```python
from build123d import *

# Parameters (mm, degrees)
F0_W      = 50
F0_H      = 12.5
F1_DEPTH  = 8
F2_DEPTH  = 75
F4_DEPTH  = 8
F7_DEPTH  = 3
F8_DEPTH  = 1
F11_DEPTH = 3
F14_DEPTH = 3
F15_DEPTH = 8
F16_DEPTH = 8
F17_DEPTH = 12.5
F18_DEPTH = 8


# Not quite as in the source:
# - a feature names something its author has since deleted; it is built from what else it names


with BuildPart() as f1:
    # F0 (on Top) → F1 (new body)
    with BuildSketch(Plane.XY):
        Polygon((42.0179491924, -72.7772228311), (84.0358983849, 0), (42.0179491924, 72.7772228311), (-42.0179491924, 72.7772228311), (-84.0358983849, 0), (-42.0179491924, -72.7772228311), align=None)
        with Locations((0, 54.5829171234)):
            Rectangle(F0_W, F0_H, mode=Mode.SUBTRACT)
    extrude(amount=F1_DEPTH)

    # F0 (on Top) → F2 (join)
    with BuildSketch(Plane.XY):
        Polygon((67.6939940411, -34.3050086158), (87.5, 0), (84.0358983849, 0), (42.0179491924, -72.7772228311), (-42.0179491924, -72.7772228311), (-84.0358983849, 0), (-87.5, 0), (-43.75, -75.7772228311), (43.75, -75.7772228311), (63.1939940411, -42.0992372499), align=None)
    extrude(amount=F2_DEPTH)

    # F0 (on Top) → F4 (join)
    with BuildSketch(Plane.XY):
        Polygon((43.75, 75.7772228311), (-43.75, 75.7772228311), (-65.625, 37.8886114156), (-68.125, 33.5584843966), (-87.5, 0), (-84.0358983849, 0), (-42.0179491924, 72.7772228311), (42.0179491924, 72.7772228311), (84.0358983849, 0), (87.5, 0), align=None)
    extrude(amount=F4_DEPTH)

    # F6 (on face) → F7 (join)
    with BuildSketch(Plane(origin=(0, -50.1312366318, 89.3836679776), x_dir=(1, 0, 0), z_dir=(0, 0.4891706574, -0.872188092))):
        Polygon((43.75, 29.4041920927), (0, 29.4041920927), (-43.75, 29.4041920927), (-42.01795, -57.4775522498), (42.01795, -57.4775522498), align=None)
    extrude(amount=F7_DEPTH)

    # F3 (on Front) → F8 (join)
    with BuildSketch(Plane.XZ):
        Polygon((-42.01795, 114.5), (0, 114.5), (42.01795, 114.5), (84.0359, 75), (87.5, 75), (42.01795, 117.5), (0, 117.5), (-42.01795, 117.5), (-87.5, 75), (-84.0359, 75), align=None)
    extrude(amount=F8_DEPTH)

    # F10 (on face) → F11 (join)
    with BuildSketch(Plane(origin=(-67.6846727043, -39.0777640058, 72.4338274863), x_dir=(0.7723629594, -0.3015876344, 0.5590173143), z_dir=(-0.6351814378, -0.3667221741, 0.6797495039))):
        Polygon((33.2314262259, 55.789645187), (-25.6554603702, 35.6104118215), (30.9888924807, -31.0804218073), align=None)
    extrude(amount=-F11_DEPTH)

    # F13 (on face) → F14 (join)
    with BuildSketch(Plane(origin=(67.6756688636, -39.5950852503, 72.4241918832), x_dir=(0.7733047167, 0.3041472681, -0.556322078), z_dir=(-0.6340345536, 0.3709553614, -0.6785221475))):
        Polygon((-30.939509805, 30.5117392321), (-32.8751652468, -56.3649154418), (25.9400068576, -35.9776056011), align=None)
    extrude(amount=F14_DEPTH)

    # F0 (on Top) → F15 (join)
    with BuildSketch(Plane.XY):
        with Locations((0, 54.5829171234)):
            Rectangle(F0_W, F0_H)
    extrude(amount=F15_DEPTH)

    # F0 (on Top) → F16 (join)
    with BuildSketch(Plane.XY):
        Polygon((75.395275497, -33.566783298), (73.1502941936, -37.4552049777), (77.4800811039, -39.9550086158), (79.6937291893, -36.1208576617), align=None)
        Polygon((73.1502941936, -37.4552049777), (67.6939940411, -34.3050086158), (63.1939940411, -42.0992372499), (68.6500615294, -45.249299283), (72.9800811039, -47.7492372499), (77.4800811039, -39.9550086158), align=None)
    extrude(amount=F16_DEPTH)

    # F0 (on Top) → F17 (cut, symmetric)
    with BuildSketch(Plane.XY):
        with Locations((0, 54.5829171234)):
            Rectangle(F0_W, F0_H)
    extrude(amount=F17_DEPTH, both=True, mode=Mode.SUBTRACT)

    # F0 (on Top) → F18 (join)
    with BuildSketch(Plane.XY):
        Polygon((72.9800811039, -47.7492372499), (68.6500615294, -45.249299283), (66.405071243, -49.1377365216), (70.7174794095, -51.6681783419), align=None)
    extrude(amount=F18_DEPTH)


solid = f1.part
```
Could you check a few things on this model? Use its own coordinates, in mm. A direction names the side the tool comes from. Give positions to 0.01 mm unless a question says otherwise; leave off trailing zeros. Loops run counter-clockwise (first coordinate to the right, second up) from the corner with the lowest first, then second, coordinate; pieces in that order, holes last. Notation, with made-up numbers: (83.25, 83) -> (102.25, 83) arc R30 cw to (102.25, 119) -> close; hole circle Ø4 at (53.5, 30). An arc over 180 degrees is marked (long way). Put each result on its own line as item: value.
(1) Please list where these lines run through material, in increasing order: probe 1 along Z at (x, y) = (-24, 3); probe 2 along X at (y, z) = (-29.5, 59.5); probe 3 along X at (y, z) = (-30, 94.5). Write a range as [from, to].
Computed:
probe 1: [0, 8]
probe 2: [-70.47, -67], [67, 70.47]
probe 3: [-49.31, -44.59], [44.93, 49.66]
(2) Thinking about a two-plate mould opening in X: for faces 1 (the face through (54.57, -25.47, 92.39)), 2 (the face through (-25, 54, 4)), 3 (the face through (71, -40, 8)), which applies, pulls with the +X half, pulls with the -X half, needs draft (parallel to the pull), parting line crosses it, or undercut?
Computed:
face 1: pulls with the +X half
face 2: undercut
face 3: needs draft
(3) For faces 4 (the face through (68.531, -50.385, 3.944)), 5 (the face through (-54.822, -24.821, 92.145)), 6 (the face through (0, 60.833, 4)), 7 (the face through (53.532, -23.251, 90.155)), which set-ups out of +Z, -Z, +X, -X, +Y, -Y let a thin tool reach every point of the face, with its end or its side?
Computed:
face 4: +Z, -Z, -Y
face 5: +Z, -X, -Y
face 6: +Z, -Z
face 7: +Y
(4) Imagine slicing it at D-D on y = 54. Write out the boundary of the cut face in (x, z).
Computed:
outline: (-56.32, 0) -> (-25, 0) -> (-25, 8) -> (-56.32, 8) -> close; (25, 0) -> (56.32, 0) -> (56.32, 8) -> (25, 8) -> close
(5) Imagine slicing it at B-B on z = 52. Write out the boundary of the cut face in (x, y) (3 decimals).
Computed:
outline: (-87.5, 0) -> (-43.75, -75.777) -> (43.75, -75.777) -> (87.5, 0) -> (84.036, 0) -> (42.018, -72.777) -> (-42.018, -72.777) -> (-84.036, 0) -> close
(6) Imagine slicing it at A-A on y = -29.5. Write out the boundary of the cut face in (x, z), plus the area to 3 significant figures.
Computed:
outline: (-70.47, 0) -> (70.47, 0) -> (70.47, 75) -> (70.66, 75.15) -> (42.83, 101.16) -> (42.69, 100.95) -> (-42.69, 100.95) -> (-70.47, 75) -> close; hole (-67, 8) -> (67, 8) -> (67, 74.15) -> (42, 97.52) -> (-41.65, 97.52) -> (-67, 73.82) -> close
area: 2,110 mm^2
(7) Imagine slicing it at C-C on x = -38.5. Write out the boundary of the cut face in (y, z), plus the area to 3 significant figures.
Computed:
outline: (-75.78, 0) -> (75.78, 0) -> (75.78, 8) -> (-72.78, 8) -> (-72.78, 73.24) -> (1.47, 114.88) -> (0, 117.5) -> (-1, 117.5) -> (-1, 116.94) -> (-75.78, 75) -> close
area: 1,670 mm^2
(8) I'm going to push flat-ended pins straight in: pin 1 Ø1.1 at (x, y) = (10.5, -0.5) entering from +Z; pin 2 Ø1.5 at (y, z) = (1, 55) entering from +X; pin 3 Ø2.5 at (y, z) = (54, 5) entering from +X; pin 4 Ø19.5 at (x, z) = (15.5, 43.5) entering from +Y. Where does each tip first touch, or does it pass through?
Computed:
pin 1: z = 117.5
pin 2: through
pin 3: x = 57.04
pin 4: y = -72.78
